Job drawing, mm, ordinate dimensions from the low corner. One solid piece. A direction names the side the tool comes from. Coordinates: 2 decimals unless noted, no trailing zeros. Loops run counter-clockwise (first coordinate to the right, second up) from the corner with the lowest first, then second, coordinate; pieces in that order, holes last. Notation, with made-up numbers: (64, -11.5) -> (122, -11.5) arc R30 cw to (122, 25.5) -> close; hole circle Ø6 at (85, 62.25). An arc over 180 degrees is marked (long way). Use one line per item in the form item = value. Start each with the question number.
(1) Pin check, flat tips, straight feed: P1, Ø2, axis at x = 36.5, y = 37, coming from the +Z side; P2, Ø0.8, axis at x = 36.5, y = 5.5, coming from the +Z side; P3, Ø12, axis at x = 27, z = 44, coming from the +Y side (1 decimal). Stop position of each tip, or through.
(2) Band-saw the part on B-B on x = 28.5. Give the cut face in (y, z), then the cut area to 3 significant figures.
(3) 3-axis set-ups, long thin cutter, end or side, ignore diameter. For the marked faces 1 and 2: which of +Z, -Z, +X, -X, +Y, -Y reach the whole face in a straight line?
(4) Band-saw the part on C-C on z = 32. Give the cut face in (x, y).
(5) Drill centre lines: L1, parallel to Z at x = 16, y = 30; L2, parallel to Z at x = 8.5, y = 13; L3, parallel to Y at x = 21, z = 38.5 (1 decimal). Where is each one in solid material? Low to high. Write a range as [from, to].
(6) Band-saw the part on A-A on z = 5. Give the cut face in (x, y), then the cut area to 3 significant figures.
(7) Band-saw the part on D-D on y = 33.5. Give the cut face in (x, z).
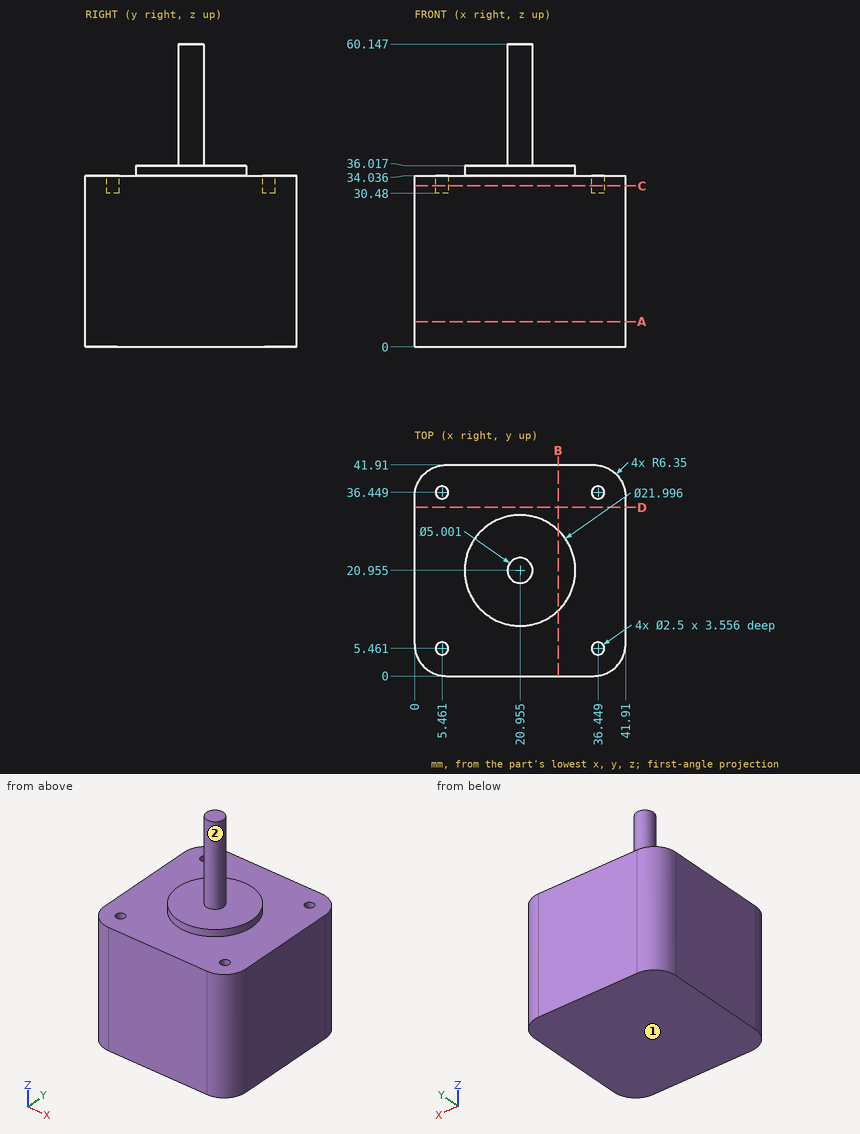
A:
q1.P1 = 34.04
q1.P2 = 30.48
q1.P3 = 23.5
q2.outline = (0, 0) -> (41.91, 0) -> (41.91, 34.04) -> (28.96, 34.04) -> (28.96, 36.02) -> (12.95, 36.02) -> (12.95, 34.04) -> (0, 34.04) -> close
q2.area = 1,460 mm²
q3.face_1 = -Z, +X, -X, +Y, -Y
q3.face_2 = +Z
q4.outline = (0, 6.35) arc R6.35 ccw to (6.35, 0) -> (35.56, 0) arc R6.35 ccw to (41.91, 6.35) -> (41.91, 35.56) arc R6.35 ccw to (35.56, 41.91) -> (6.35, 41.91) arc R6.35 ccw to (0, 35.56) -> close; hole circle Ø2.5 at (5.46, 5.46); hole circle Ø2.5 at (5.46, 36.45); hole circle Ø2.5 at (36.45, 5.46); hole circle Ø2.5 at (36.45, 36.45)
q5.L1 = [0, 36.02]
q5.L2 = [0, 34.04]
q5.L3 = [18.5, 23.5]
q6.outline = (0, 6.35) arc R6.35 ccw to (6.35, 0) -> (35.56, 0) arc R6.35 ccw to (41.91, 6.35) -> (41.91, 35.56) arc R6.35 ccw to (35.56, 41.91) -> (6.35, 41.91) arc R6.35 ccw to (0, 35.56) -> close
q6.area = 1,720 mm²
q7.outline = (0, 0) -> (41.91, 0) -> (41.91, 34.04) -> (0, 34.04) -> close
